Read the model definition and answer for the solid it produces. Units are mm, in the model's axes. A direction names the side the tool comes from. Coordinates: 2 decimals unless noted, no trailing zeros. Write each loop counter-clockwise with the first axis right and the second up, starting at its lowest first coordinate (ties: lowest second). Pieces come first, ordered by that corner, then holes.
from build123d import *

# Parameters (mm, degrees)
F0_W     = 5
F0_H     = 30
F0_W_2   = 35
F1_DEPTH = 5
F2_DEPTH = 100
F3_W     = 40
F3_H     = 30
F3_R     = 10
F4_DEPTH = 5
F5_R     = 5


with BuildPart() as f1:
    # F0 (on Top) → F1 (new body)
    with BuildSketch(Plane.XY):
        with Locations((-17.5, 0)):
            Rectangle(F0_W, F0_H)
        with Locations((2.5, 0)):
            Rectangle(F0_W_2, F0_H)
    extrude(amount=-F1_DEPTH)

    # F0 (on Top) → F2 (join)
    with BuildSketch(Plane.XY):
        with Locations((-17.5, 0)):
            Rectangle(F0_W, F0_H)
    extrude(amount=F2_DEPTH)

    # F3 (on face) → F4 (join)
    with BuildSketch(Plane.XY.offset(100)):
        Rectangle(F3_W, F3_H)
        with Locations((5, 0)):
            Circle(F3_R, mode=Mode.SUBTRACT)
    extrude(amount=F4_DEPTH)

    # F5
    f5_edges = [f1.edges().sort_by_distance(p)[0] for p in [
        (-20, 0, -5),
        (-20, 0, 105),
    ]]
    fillet(f5_edges, radius=F5_R)


solid = f1.part
Item 1: Determine the mould class of faces 1 (the flat face through (20, 0, -2)), 2 (the flat face through (-15, 0, 49)), 3 (the flat face through (2, 0, -5)), 4 (the flat face through (2, 0, 0)) for opening direction Z: +Z half, -Z half, draft (parallel to the pull), parting line (faces both ways), or undercut.
Item 2: Find the intervals of material crossed by probe 1 along Y at (x, z) = (5, 101.65); probe 2 along Z at (x, y) = (-5, -5.25); probe 3 along X at (y, z) = (1, 66.5), in increasing order.
Item 3: The part is cut by section C-C (x = 5). Give the vertices of the cut face in (y, z), and give its area (3 significant figures).
Item 4: The part is cut by section D-D (y = 11). Give the vertices of the cut face in (x, z), and give its area (3 significant figures).
Item 5: The part is cut by section A-A (x = -10). Give the vertices of the cut face in (y, z).
Item 6: Given pin 1 (8 mm diameter, centred on x = 13.5, z = 94, fed in from -Y); pin 2 (1.5 mm diameter, centred on y = -0.5, z = 67, fed in from +X); pin 3 (1.5 mm diameter, centred on x = 0, y = -4.5, fed in from +Z), each flat-ended and moving along its own axis, determine where each tip first touches the part or whether it passes through.
Item 7: The part is cut by section B-B (y = 0). Give the vertices of the cut face in (x, z), and give its area (3 significant figures).
Item 8: For faces 5 (the flat face through (-6, 0, 105)), 6 (the flat face through (-6, 0, 100)), 7 (the cylindrical face through (14.54, 3, 102.46)), determine the directions among +Z, -Z, +X, -X, +Y, -Y from which every point of the face is accessible in a straight line to the end or side of a thin tool.
Answer:
1. face 1: draft
1. face 2: undercut
1. face 3: -Z half
1. face 4: undercut
2. probe 1: y = -15 to -10, 10 to 15
2. probe 2: z = -5 to 0, 100 to 105
2. probe 3: x = -20 to -15
3. outline: (-15, -5) - (15, -5) - (15, 0) - (-15, 0) - close; (-15, 100) - (-10, 100) - (-10, 105) - (-15, 105) - close; (10, 100) - (15, 100) - (15, 105) - (10, 105) - close
3. area: 200 mm2
4. outline: (-20, 0) arc R5 ccw to (-15, -5) - (20, -5) - (20, 0) - (-15, 0) - (-15, 100) - (20, 100) - (20, 105) - (-15, 105) arc R5 ccw to (-20, 100) - close
4. area: 889 mm2
5. outline: (-15, -5) - (15, -5) - (15, 0) - (-15, 0) - close; (-15, 100) - (15, 100) - (15, 105) - (-15, 105) - close
6. pin 1: passes through
6. pin 2: stops at x = -15
6. pin 3: stops at z = 0
7. outline: (-20, 0) arc R5 ccw to (-15, -5) - (20, -5) - (20, 0) - (-15, 0) - (-15, 100) - (-5, 100) - (-5, 105) - (-15, 105) arc R5 ccw to (-20, 100) - close; (15, 100) - (20, 100) - (20, 105) - (15, 105) - close
7. area: 789 mm2
8. face 5: +Z, +X, -X, +Y, -Y
8. face 6: +X, +Y, -Y
8. face 7: +Z
